CAD build for the part. Positions are in the model's coordinates, mm. A direction names the side the tool comes from. Round coordinates to 2 decimals unless told otherwise and drop trailing zeros. Loops run counter-clockwise (first coordinate to the right, second up) from the corner with the lowest first, then second, coordinate; pieces in that order, holes last. Notation, with made-up numbers: M 23.5,20 L 76.5,20 A27 ccw 76.5,53 Z; hole C 17,67.25 d6. An arc over 180 degrees is marked long. Use a Markdown table: item, result. Add a question column.
(1) Flat gauge pins, fed straight in: P1, Ø6.5, axis at x = 38, z = 8, coming from the +Y side; P2, Ø8, axis at x = 5, z = 6.5, coming from the +Y side; P3, Ø1, axis at y = 12, z = 5.5, coming from the -X side. Where does each tip first touch, or does it go through?
(2) Band-saw the part on C-C, the plane x = 5. Write the cut outline in (y, z), and give its area (3 significant figures).
(3) Which spindle directions (+Z, -Z, +X, -X, +Y, -Y) get a long thin tool onto all of the face, cutting with end or side? Do faces 1 (the face through (20, 11, 15)), 2 (the face through (3, 5, 8)), 3 (the face through (37, 5, 8)). Say none if no direction does.
(4) Band-saw the part on B-B, the plane y = 2.5. Write the cut outline in (x, z).
(5) Wall check: L1, parallel to Y at x = 35, z = 3; L2, parallel to X at y = 6.5, z = 6; L3, parallel to X at y = 7.5, z = 1. Give the ranges that are in metal, low to high.
(6) Band-saw the part on D-D, the plane y = 10.5. Write the cut outline in (x, z).
(7) Band-saw the part on A-A, the plane z = 2.75. Write the cut outline in (x, y), and give its area (3 significant figures).
from build123d import *

# Parameters (mm, degrees)
CROQUIS1_W              = 40
CROQUIS1_H              = 15
SALIENTE_EXTRUIR1_DEPTH = 15
CROQUIS2_W              = 10
CROQUIS2_H              = 10
CORTAR_EXTRUIR2_DEPTH   = 15
CORTAR_EXTRUIR3_DEPTH   = 15
CORTAR_EXTRUIR4_DEPTH   = 15
SALIENTE_EXTRUIR2_DEPTH = 15


with BuildPart() as part:
    # Croquis1 → Saliente-Extruir1 (new body)
    with BuildSketch(Plane(origin=(0, 0, 0), x_dir=(1, 0, 0), z_dir=(0, 1, 0))):
        with Locations((20, -7.5)):
            Rectangle(CROQUIS1_W, CROQUIS1_H)
    extrude(amount=SALIENTE_EXTRUIR1_DEPTH)

    # Croquis2 → Cortar-Extruir2 (cut)
    with BuildSketch(Plane.XY.offset(15)):
        with Locations((5, 10)):
            Rectangle(CROQUIS2_W, CROQUIS2_H)
        with Locations((35, 10)):
            Rectangle(CROQUIS2_W, CROQUIS2_H)
    extrude(amount=-CORTAR_EXTRUIR2_DEPTH, mode=Mode.SUBTRACT)

    # Croquis5 → Cortar-Extruir3 (cut)
    with BuildSketch(Plane.XY.offset(15)):
        with BuildLine():
            ThreePointArc((30, 0), (20, 10), (10, 0))
            Line((10, 0), (30, 0))
        make_face()
        with BuildLine():
            Line((30, 0), (10, 0))
            ThreePointArc((10, 0), (20, -10), (30, 0))
        make_face()
    extrude(amount=-CORTAR_EXTRUIR3_DEPTH, mode=Mode.SUBTRACT)

    # Croquis6 → Cortar-Extruir4 (cut)
    with BuildSketch(Plane.XY.offset(15)):
        with BuildLine():
            Line((20, 15), (10, 15))
            Line((10, 15), (10, 11.180339887))
            ThreePointArc((10, 11.180339887), (14.647668653, 14.012585384), (20, 15))
        make_face()
        with BuildLine():
            Line((30, 15), (20, 15))
            ThreePointArc((20, 15), (25.352331347, 14.012585384), (30, 11.180339887))
            Line((30, 11.180339887), (30, 15))
        make_face()
    extrude(amount=-CORTAR_EXTRUIR4_DEPTH, mode=Mode.SUBTRACT)

    # Croquis7 → Saliente-Extruir2 (add)
    with BuildSketch(Plane.XY.offset(15)):
        with BuildLine():
            ThreePointArc((10, 11.180339887), (7.539669812, 8.351058113), (5.857864376, 5))
            Line((5.857864376, 5), (10, 5))
            Line((10, 5), (10, 11.180339887))
        make_face()
        with BuildLine():
            Line((30, 5), (34.142135624, 5))
            ThreePointArc((34.142135624, 5), (32.460330188, 8.351058113), (30, 11.180339887))
            Line((30, 11.180339887), (30, 5))
        make_face()
    extrude(amount=-SALIENTE_EXTRUIR2_DEPTH)


solid = part.part
Return value:
| question | item | result |
|---|---|---|
| 1 | P1 | y = 5 |
| 1 | P2 | y = 10.2 |
| 1 | P3 | x = 10.37 |
| 2 | outline | M 0,0 L 5,0 L 5,15 L 0,15 Z |
| 2 | area | 75.0 mm^2 |
| 3 | face 1 | +Z, +X, -X, +Y, -Y |
| 3 | face 2 | +Z, -Z, -X, +Y |
| 3 | face 3 | +Z, -Z, +X, +Y |
| 4 | outline | M 0,0 L 10.32,0 L 10.32,15 L 0,15 Z; M 29.68,0 L 40,0 L 40,15 L 29.68,15 Z |
| 5 | L1 | 0 to 5 |
| 5 | L2 | 6.48 to 12.4, 27.6 to 33.52 |
| 5 | L3 | 7.01 to 13.39, 26.61 to 32.99 |
| 6 | outline | M 9.29,0 L 30.71,0 L 30.71,15 L 9.29,15 Z |
| 7 | outline | M 0,0 L 10,0 A10 cw 30,0 L 40,0 L 40,5 L 34.14,5 A15 ccw 5.86,5 L 0,5 Z |
| 7 | area | 249 mm^2 |
